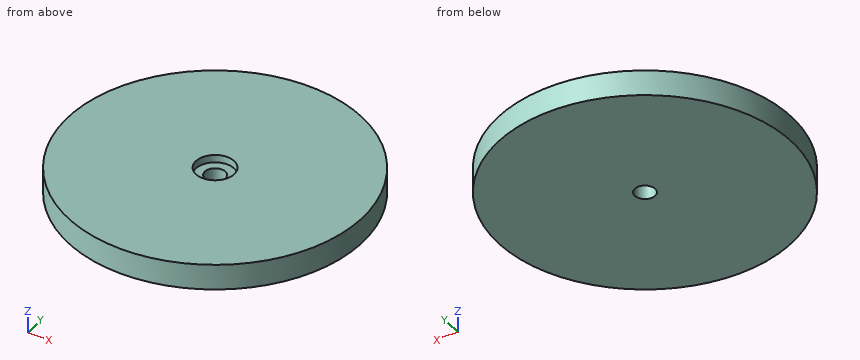
from build123d import *

# Parameters (mm, degrees)
SKETCH1_R           = 57.5
BOSS_EXTRUDE1_DEPTH = 10
SKETCH2_R           = 7.5
SKETCH2_R_2         = 4
CUT_EXTRUDE1_DEPTH  = 3
SKETCH2_2_R         = 4
CUT_EXTRUDE2_DEPTH  = 82.929848041


with BuildPart() as part:
    # Sketch1 → Boss-Extrude1 (new body)
    with BuildSketch(Plane.XY):
        Circle(SKETCH1_R)
    extrude(amount=BOSS_EXTRUDE1_DEPTH)

    # Sketch2 → Cut-Extrude1 (cut)
    with BuildSketch(Plane.XY.offset(10)):
        Circle(SKETCH2_R)
        Circle(SKETCH2_R_2, mode=Mode.SUBTRACT)
    extrude(amount=-CUT_EXTRUDE1_DEPTH, mode=Mode.SUBTRACT)

    # Sketch2<2> → Cut-Extrude2 (cut, through all)
    with BuildSketch(Plane.XY.offset(10)):
        Circle(SKETCH2_2_R)
    extrude(amount=-CUT_EXTRUDE2_DEPTH, mode=Mode.SUBTRACT)


solid = part.part
Verification items for the finished model (mm, model axes). Give positions to 0.01 mm unless a question says otherwise; leave off trailing zeros. Loops run counter-clockwise (first coordinate to the right, second up) from the corner with the lowest first, then second, coordinate; pieces in that order, holes last. Notation, with made-up numbers: (27.5, 40) - (69.5, 40) arc R18 ccw to (69.5, 61) - close; hole circle Ø6 at (24.25, 8). An arc over 180 degrees is marked (long way). Write item = value, one per line. Start each with the question number.
Q1. Cross-section at A-A, the plane y = 0. Enter the section's corners in (x, z), and give its area (3 significant figures).
Q2. Cross-section at D-D, the plane x = 16.5. Enter the section's corners in (y, z), and give its area (3 significant figures).
Q3. Cross-section at C-C, the plane z = 1.5. Enter the section's corners in (x, y), and give its area (3 significant figures).
Q4. Depth check by flat-ended pin: P1, Ø5, axis at x = 26, z = 2, coming from the -Y side; P2, Ø5, axis at y = 33.5, z = 4, coming from the +X side; P3, Ø5, axis at x = 0, y = 0, coming from the -Z side; P4, Ø3, axis at y = -9.5, z = 6, coming from the +X side. Enter the tip coordinate at first touch or a pass-through.
Q5. Thickness scan on line 1 (Y direction, x = 0, z = 2.5); line 2 (Y direction, x = 0, z = 7.85); line 3 (X direction, y = 2.5, z = 9). Record the ranges inside material, lowest first.
Answer key:
q1.outline = (-57.5, 0) - (-4, 0) - (-4, 7) - (-7.5, 7) - (-7.5, 10) - (-57.5, 10) - close; (4, 0) - (57.5, 0) - (57.5, 10) - (7.5, 10) - (7.5, 7) - (4, 7) - close
q1.area = 1,050 mm^2
q2.outline = (-55.08, 0) - (55.08, 0) - (55.08, 10) - (-55.08, 10) - close
q2.area = 1,100 mm^2
q3.outline = circle Ø115 at (0, 0); hole circle Ø8 at (0, 0)
q3.area = 10,300 mm^2
q4.P1 = -52.48
q4.P2 = 48.43
q4.P3 = through
q4.P4 = 56.94
q5.line_1 = -57.5 to -4, 4 to 57.5
q5.line_2 = -57.5 to -7.5, 7.5 to 57.5
q5.line_3 = -57.45 to -7.07, 7.07 to 57.45
